```python
from build123d import *

# Parameters (mm, degrees)
F0_R     = 1.5
F1_DEPTH = 2.8


with BuildPart() as f1:
    # F0 (on Top) → F1 (new body)
    with BuildSketch(Plane.XY):
        with BuildLine():
            ThreePointArc((-3.746999, -1.4), (-4, 0), (-3.746999, 1.4))
            Line((-3.746999, 1.4), (-6.546999, 1.4))
            Line((-6.546999, 1.4), (-6.546999, -1.4))
            Line((-6.546999, -1.4), (-3.746999, -1.4))
        make_face()
        with BuildLine():
            Line((3.746999, -1.4), (3.746999, 1.4))
            ThreePointArc((3.746999, 1.4), (0, 4), (-3.746999, 1.4))
            Line((-3.746999, 1.4), (-3.746999, -1.4))
            ThreePointArc((-3.746999, -1.4), (0, -4), (3.746999, -1.4))
        make_face()
        Circle(F0_R, mode=Mode.SUBTRACT)
        with BuildLine():
            Line((-3.746999, -1.4), (-3.746999, 1.4))
            ThreePointArc((-3.746999, 1.4), (-4, 0), (-3.746999, -1.4))
        make_face()
        with BuildLine():
            ThreePointArc((3.746999, 1.4), (3.936242, 0.711338), (4, 0))
            ThreePointArc((4, 0), (3.936242, -0.711338), (3.746999, -1.4))
            Line((3.746999, -1.4), (6.546999, -1.4))
            Line((6.546999, -1.4), (6.546999, 1.4))
            Line((6.546999, 1.4), (3.746999, 1.4))
        make_face()
        with BuildLine():
            ThreePointArc((3.746999, -1.4), (3.936242, -0.711338), (4, 0))
            ThreePointArc((4, 0), (3.936242, 0.711338), (3.746999, 1.4))
            Line((3.746999, 1.4), (3.746999, -1.4))
        make_face()
    extrude(amount=F1_DEPTH)


solid = f1.part
```
Here's how the part is built. I have some questions about the finished solid (model axes, mm). A direction names the side the tool comes from. Round coordinates to 2 decimals unless told otherwise and drop trailing zeros. Loops run counter-clockwise (first coordinate to the right, second up) from the corner with the lowest first, then second, coordinate; pieces in that order, holes last. Notation, with made-up numbers: (69.25, 59) -> (123.25, 59) arc R8 ccw to (123.25, 73) -> close; hole circle Ø1 at (55.25, 45). An arc over 180 degrees is marked (long way). Answer as CSV lines item,"result". Start each with the question number.
1. For faces 4 (the face through (-2, 0, 0)), 5 (the face through (5, 1.4, 1)), 6 (the face through (-5, -1.4, 1)), 7 (the face through (0, 4, 1)), 8 (the face through (5, -1.4, 1)), which set-ups out of +Z, -Z, +X, -X, +Y, -Y let a thin tool reach every point of the face, with its end or its side?
2. Imagine slicing it at B-B on y = 0. Write out the boundary of the cut face in (x, z).
3. If we mould it in two halves opening along X, with no side actions, what happens to faces 1 (the face through (-1.5, 0.07, 1.38)), 2 (the face through (0, -4, 1)), 3 (the face through (-5, 1.4, 1))? For each: pulls with the +X half, pulls with the -X half, needs draft (parallel to the pull), parting line crosses it, or undercut.
4. I need wall thicknesses on probe 1 along Y at (x, z) = (0, 2.25); probe 2 along Y at (x, z) = (4.75, 2.15); probe 3 along Y at (x, z) = (1, 0.2). Which ranges of each line are inside material? Lowest first, please. Write a range as from..to.
5. Imagine slicing it at A-A on x = 0. Write out the boundary of the cut face in (y, z), plus the area to 3 significant figures.
6. Imagine slicing it at D-D on y = -2. Write out the boundary of the cut face in (x, z).
7. Imagine slicing it at C-C on z = 0.9. Write out the boundary of the cut face in (x, y).
8. I'm going to push flat-ended pins straight in: P1, Ø0.8, axis at x = 4.5, z = 2, coming from the +Y side; P2, Ø1.5, axis at x = -3, y = -3, coming from the -Z side; P3, Ø1, axis at x = 4, z = 1, coming from the +Y side. Where does each tip first touch, or does it pass through?
Solution:
1,face 4,"-Z, +X, -X, +Y, -Y"
1,face 5,"+Z, -Z, +X, +Y"
1,face 6,"+Z, -Z, -X, -Y"
1,face 7,"+Z, -Z, +Y"
1,face 8,"+Z, -Z, +X, -Y"
2,outline,"(-6.55, 0) -> (-1.5, 0) -> (-1.5, 2.8) -> (-6.55, 2.8) -> close; (1.5, 0) -> (6.55, 0) -> (6.55, 2.8) -> (1.5, 2.8) -> close"
3,face 1,"undercut"
3,face 2,"parting line crosses it"
3,face 3,"needs draft"
4,probe 1,"-4..-1.5, 1.5..4"
4,probe 2,"-1.4..1.4"
4,probe 3,"-3.87..-1.12, 1.12..3.87"
5,outline,"(-4, 0) -> (-1.5, 0) -> (-1.5, 2.8) -> (-4, 2.8) -> close; (1.5, 0) -> (4, 0) -> (4, 2.8) -> (1.5, 2.8) -> close"
5,area,"14.0 mm²"
6,outline,"(-3.46, 0) -> (3.46, 0) -> (3.46, 2.8) -> (-3.46, 2.8) -> close"
7,outline,"(-6.55, -1.4) -> (-3.75, -1.4) arc R4 ccw to (3.75, -1.4) -> (6.55, -1.4) -> (6.55, 1.4) -> (3.75, 1.4) arc R4 ccw to (-3.75, 1.4) -> (-6.55, 1.4) -> close; hole circle Ø3 at (0, 0)"
8,P1,"y = 1.4"
8,P2,"z = 0"
8,P3,"y = 1.94"
